Read the model definition and answer for the solid it produces. Units are mm, in the model's axes. A direction names the side the tool comes from. Coordinates: 2 decimals unless noted, no trailing zeros. Order: outer loops, then holes, each group sorted by start corner. A loop starts at its lowest first (then second) coordinate and runs counter-clockwise, first axis right, second up. Notation, with made-up numbers: (-34.5, 80.5) -> (-11.5, 80.5) arc R12 ccw to (-11.5, 97.5) -> close; hole circle Ø10 at (-33, 71.25). An arc over 180 degrees is marked (long way). Return JSON: item names as keys, results as strings. Group by question number.
```python
from build123d import *

# Parameters (mm, degrees)
F0_W     = 1150
F0_H     = 650
F1_DEPTH = 725
F2_W     = 180
F2_H     = 495
F3_DEPTH = 650.001
F5_DEPTH = 650.001
F6_W     = 910
F6_H     = 160
F7_DEPTH = 380


with BuildPart() as f1:
    # F0 (on Top) → F1 (new body)
    with BuildSketch(Plane.XY):
        with Locations((-575, -14.591489)):
            Rectangle(F0_W, F0_H)
    extrude(amount=F1_DEPTH)

    # F2 (on face) → F3 (cut, through all)
    with BuildSketch(Plane.XZ.offset(339.591489)):
        with Locations((-110, 457.5)):
            Rectangle(F2_W, F2_H)
    extrude(amount=-F3_DEPTH, mode=Mode.SUBTRACT)

    # F4 (on face) → F5 (cut, through all)
    with BuildSketch(Plane.XZ.offset(339.591489)):
        Polygon((-220, 545), (-712.675017, 545), (-712.675017, 0), (-220, 0), (-20, 0), (-20, 190), (-220, 190), align=None)
    extrude(amount=-F5_DEPTH, mode=Mode.SUBTRACT)

    # F6 (on face) → F7 (cut)
    with BuildSketch(Plane.XZ.offset(339.591489)):
        with Locations((-675, 625)):
            Rectangle(F6_W, F6_H)
    extrude(amount=-F7_DEPTH, mode=Mode.SUBTRACT)


solid = f1.part
```
1. Given pin 1 (4 mm diameter, centred on x = -442.5, y = 197.5, fed in from -Z), flat-ended and moving along its own axis, determine where the tip first touches the part or whether it passes through.
2. Find section C-C on y = 251. Determine the outline of the cut face in (x, z).
3. Straight lines are drawn through the part: L1, parallel to X at y = 152, z = 457; L2, parallel to X at y = -257, z = 602.5; L3, parallel to X at y = -127, z = 99. For each, find the intervals that lie inside material, in ascending order.
4. For a pull along Z with two mould halves and no side action, classify faces 6 (the face through (-583, -10, 725)), 7 (the face through (-200, -19, 454)), 8 (the face through (0, -19, 357)) as released by +Z, released by -Z, zero draft, split by the parting line, or undercut.
5. Find section A-A on x = -183.5. Determine the outline of the cut face in (y, z).
6. Find section D-D on z = 241.5. Determine the outline of the cut face in (x, y), and give its area (3 significant figures).
7. Which of the six approach directions +Z, -Z, +X, -X, +Y, -Y give full straight-line access (tool end or side, diameter ignored) to faces 1 (the face through (-1130, -152, 624)), 2 (the face through (-111, -19, 210)), 3 (the face through (-20, -19, 94)), 4 (the face through (-220, -19, 387)), 5 (the face through (-1150, -19, 357))?
8. Find section B-B on z = 76.5. Determine the outline of the cut face in (x, y), and give its area (3 significant figures).
Result:
{
 "1": {"pin 1": "z = 545"},
 "2": {"outline": "(-1150, 0) -> (-712.68, 0) -> (-712.68, 545) -> (-220, 545) -> (-220, 190) -> (-20, 190) -> (-20, 0) -> (0, 0) -> (0, 725) -> (-1150, 725) -> close; hole (-200, 210) -> (-20, 210) -> (-20, 705) -> (-200, 705) -> close"},
 "3": {"L1": "-1150 to -712.68, -220 to -200, -20 to 0", "L2": "-1150 to -1130, -220 to -200, -20 to 0", "L3": "-1150 to -712.68, -20 to 0"},
 "4": {"face 6": "released by +Z", "face 7": "undercut", "face 8": "zero draft"},
 "5": {"outline": "(-339.59, 190) -> (310.41, 190) -> (310.41, 210) -> (-339.59, 210) -> close; (-339.59, 705) -> (310.41, 705) -> (310.41, 725) -> (-339.59, 725) -> close"},
 "6": {"outline": "(-1150, -339.59) -> (-712.68, -339.59) -> (-712.68, 310.41) -> (-1150, 310.41) -> close; (-220, -339.59) -> (-200, -339.59) -> (-200, 310.41) -> (-220, 310.41) -> close; (-20, -339.59) -> (0, -339.59) -> (0, 310.41) -> (-20, 310.41) -> close", "area": "310,000 mm^2"},
 "7": {"face 1": "-Y", "face 2": "+Y, -Y", "face 3": "-Z, +Y, -Y", "face 4": "-Z, -Y", "face 5": "+Z, -Z, -X, +Y, -Y"},
 "8": {"outline": "(-1150, -339.59) -> (-712.68, -339.59) -> (-712.68, 310.41) -> (-1150, 310.41) -> close; (-20, -339.59) -> (0, -339.59) -> (0, 310.41) -> (-20, 310.41) -> close", "area": "297,000 mm^2"}
}
